from build123d import *

# Parameters (mm, degrees)
BOSS_EXTRUDE1_DEPTH = 4
SKETCH2_R           = 4.5
BOSS_EXTRUDE2_DEPTH = 2
SKETCH3_R           = 4.5
SKETCH3_R_2         = 3.05
BOSS_EXTRUDE3_DEPTH = 3
SKETCH4_W           = 0.8
SKETCH4_H           = 3
CUT_EXTRUDE1_DEPTH  = 5


with BuildPart() as part:
    # Sketch1 → Boss-Extrude1 (new body)
    with BuildSketch(Plane.YZ):
        Polygon((1.703183294, -2.95), (3.406366588, 0), (1.703183294, 2.95), (-1.703183294, 2.95), (-3.406366588, 0), (-1.703183294, -2.95), align=None)
    extrude(amount=BOSS_EXTRUDE1_DEPTH)

    # Sketch2 → Boss-Extrude2 (add)
    with BuildSketch(Plane.YZ.offset(4)):
        with Locations(Location((0, 0, 0), (0, 0, 270))):
            Circle(SKETCH2_R)
    extrude(amount=BOSS_EXTRUDE2_DEPTH)

    # Sketch3 → Boss-Extrude3 (add)
    with BuildSketch(Plane.YZ.offset(6)):
        with Locations(Location((0, 0, 0), (0, 0, 270))):
            Circle(SKETCH3_R)
        with Locations(Location((0, 0, 0), (0, 0, 270))):
            Circle(SKETCH3_R_2, mode=Mode.SUBTRACT)
    extrude(amount=BOSS_EXTRUDE3_DEPTH)

    # Sketch4 → Cut-Extrude1 (cut, symmetric)
    with BuildSketch(Plane(origin=(0, 0, 0), x_dir=(0, 1, 0), z_dir=(0, 0, 1))):
        with Locations((0, -7.5)):
            Rectangle(SKETCH4_W, SKETCH4_H)
    extrude(amount=CUT_EXTRUDE1_DEPTH, both=True, mode=Mode.SUBTRACT)


solid = part.part
Can you work these out from the model? Positions are in its coordinate system, mm. A direction names the side the tool comes from. Round coordinates to 2 decimals unless told otherwise and drop trailing zeros. Write each loop counter-clockwise with the first axis right and the second up, starting at its lowest first coordinate (ties: lowest second). Pieces come first, ordered by that corner, then holes. Notation, with made-up numbers: (78, 2.25) -> (105, 2.25) arc R15 cw to (105, 29.25) -> close; hole circle Ø8 at (-19.5, -1.5). An arc over 180 degrees is marked (long way). Use one line per item in the form item = value. Start each with the question number.
Q1. If I drill on probe 1 along X at (y, z) = (-2, -2); probe 2 along Y at (x, z) = (6.5, 3.5); probe 3 along Z at (x, y) = (7.5, -2), over which ranges is the centre line in solid material (lowest first)? Write a range as [from, to].
Q2. I'm going to push flat-ended pins straight in: P1, Ø4, axis at x = 6.5, z = -3.5, coming from the +Y side; P2, Ø1.2, axis at x = 8, z = -3.5, coming from the -Y side; P3, Ø1, axis at x = 2.5, y = 0.5, coming from the +Z side. Where does each tip first touch, or does it pass through?
Q3. Imagine slicing it at A-A (x = 7.75). Please give me the cut outline in (y, z), then the cut area to 3 significant figures.
Q4. Imagine slicing it at D-D (z = -0.5). Please give me the cut outline in (x, y), then the cut area to 3 significant figures.
Q5. Imagine slicing it at B-B (y = 0). Please give me the cut outline in (x, z).
Q6. Imagine slicing it at C-C (x = 3.75). Please give me the cut outline in (y, z).
Q7. Which directions (+Z, -Z, +X, -X, +Y, -Y) give clear straight access to the entire face, cutting with the end or side of a thin tool? Please do faces 1 (the face through (1.97, -2.54, 1.5)), 2 (the face through (4, 3.1, 1.1)), 3 (the face through (8, -0.4, -4)).
Q8. We'd pull the mould along Y, two halves only. Please class faces 4 (the face through (2, 0, -2.95)), 5 (the face through (7.48, 3.05, -0.06)), 6 (the face through (1.97, -2.57, -1.45)): +Y half, -Y half, draft (parallel to the pull), parting line (faces both ways), or undercut.
Worked out:
q1.probe_1 = [0, 6]
q1.probe_2 = [-2.83, -0.4], [0.4, 2.83]
q1.probe_3 = [-4.03, -2.3], [2.3, 4.03]
q2.P1 = 4.24
q2.P2 = -3.44
q2.P3 = 2.95
q3.outline = (-0.4, -4.48) -> (-0.4, -3.02) arc R3.05 cw to (-0.4, 3.02) -> (-0.4, 4.48) arc R4.5 ccw to start; (0.4, -4.48) arc R4.5 ccw to (0.4, 4.48) -> (0.4, 3.02) arc R3.05 cw to (0.4, -3.02) -> close
q3.area = 32.1 mm^2
q4.outline = (0, -3.12) -> (4, -3.12) -> (4, -4.47) -> (9, -4.47) -> (9, -3.01) -> (6, -3.01) -> (6, 3.01) -> (9, 3.01) -> (9, 4.47) -> (4, 4.47) -> (4, 3.12) -> (0, 3.12) -> close
q4.area = 51.6 mm^2
q5.outline = (0, -2.95) -> (4, -2.95) -> (4, -4.5) -> (6, -4.5) -> (6, 4.5) -> (4, 4.5) -> (4, 2.95) -> (0, 2.95) -> close
q6.outline = (-3.41, 0) -> (-1.7, -2.95) -> (1.7, -2.95) -> (3.41, 0) -> (1.7, 2.95) -> (-1.7, 2.95) -> close
q7.face_1 = +Z, -X, -Y
q7.face_2 = -X
q7.face_3 = +Z, -Z, +X
q8.face_4 = draft
q8.face_5 = undercut
q8.face_6 = -Y half
